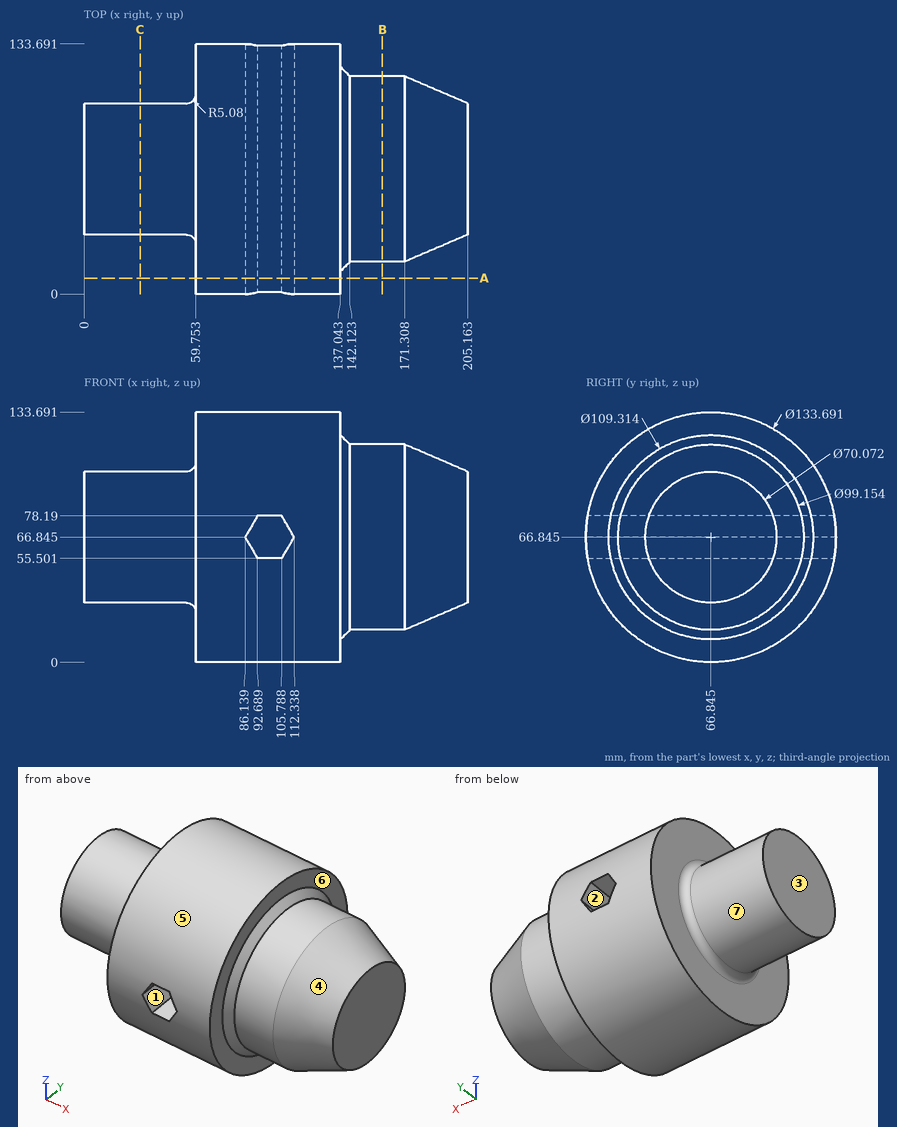
Could you check a few things on this drawing? It's one solid part, dimensions in mm from its lowest x, y, z. A direction names the side the tool comes from. Coordinates: 2 decimals unless noted, no trailing zeros. Order: outer loops, then holes, each group sorted by start corner. A loop starts at its lowest first (then second) coordinate and runs counter-clockwise, first axis right, second up. Notation, with made-up numbers: M 59,28.5 L 66,28.5 A26 cw 66,46.5 Z; hole C 19.5,20 d8. An arc over 180 degrees is marked long. Use one line per item in the form item = value. Start each with the question number.
1. Suppose I cut it at B-B on x = 159.5. Write out the boundary of the cut face in (y, z) (1 decimal).
2. For pin 1 (5 mm diameter, centred on x = 59.5, y = 102.5, fed in from +Z); pin 2 (10 mm diameter, centred on x = 99.5, z = 49, fed in from -Y); pin 3 (4 mm diameter, centred on x = 73.5, y = 63.5, fed in from +Z); pin 4 (6.5 mm diameter, centred on x = 98, y = 66, fed in from -Z), each with a flat end and sliding along its axis, tell me the tip position at first contact or that it passes through.
3. We'd pull the mould along Z, two halves only. Please class the marked faces 1, 2, 3 and 4: +Z half, -Z half, draft (parallel to the pull), parting line (faces both ways), or undercut.
4. Please list where these lines run through material, in increasing order: line 1 (X direction, y = 34, z = 63) (1 decimal); line 2 (X direction, y = 55.5, z = 71) (1 decimal); line 3 (Z direction, x = 107.5, y = 50) (1 decimal).
5. On a 3-axis mill with a long thin cutter (end or side, diameter ignored), from which of +Z, -Z, +X, -X, +Y, -Y can I reach the whole of each face in a straight line? I mean the marked faces 5, 6 and 7. Say none if no direction works.
6. Suppose I cut it at A-A on y = 8.5. Write out the boundary of the cut face in (x, z) (1 decimal), then the cut area to 3 significant figures.
7. Suppose I cut it at C-C on x = 30. Write out the boundary of the cut face in (y, z) (1 decimal).
Geometry says:
q1.outline = C 66.8,66.8 d99.2
q2.pin_1 = 124.88
q2.pin_2 = 1.25
q2.pin_3 = 133.68
q2.pin_4 = 0
q3.face_1 = undercut
q3.face_2 = undercut
q3.face_3 = draft
q3.face_4 = parting line
q4.line_1 = 0 to 88.4, 110.1 to 205.2
q4.line_2 = 0 to 88.5, 109.9 to 205.2
q4.line_3 = 2.2 to 58.5, 75.2 to 131.5
q5.face_5 = +X, -X
q5.face_6 = +X
q5.face_7 = -X
q6.outline = M 59.8,34.2 L 137,34.2 L 137,99.5 L 59.8,99.5 Z; hole M 86.1,66.8 L 92.7,55.5 L 105.8,55.5 L 112.3,66.8 L 105.8,78.2 L 92.7,78.2 Z
q6.area = 4,600 mm^2
q7.outline = C 66.8,66.8 d70.1
